Autodesk Fusion 360 part; units mm, degrees
sketch "Sketch1" plane through (0, 0, 0) normal (1, 0, 0) x (0, 1, 0)
  line L0 (0, 0) -> (15, 0) construction
  line L1 (15, 0) -> (15, 4.5) construction
  circle A0 centre (15, 4.5) radius 3
  line L2 (15, 0) -> (11, 0) construction
  line L3 (11, 0) -> (19, 0)
  line L4 (19, 0) -> (19, 3.75)
  line L5 (19, 3.75) -> (11, 3.75)
  line L6 (11, 3.75) -> (2.6, 3.75)
  line L7 (2.6, 3.75) -> (2.6, 0)
  line L8 (2.6, 0) -> (11, 0)
  dimension "d1" = 15
  dimension "d2" = 4.5
  dimension "d3" = 6
  dimension "d4" = 4
  dimension "d5" = 8
  dimension "d6" = 3.75
  dimension "d7" = 2.6
revolve "Revolve1" add sketch "Sketch1" angle 360 about axis through (0, 0, 1.75) along (0, 0, 1) contours A0 L3 L4 L5 L6 L7 L8
fillet "Fillet1" radius 1.5 1 edges at (-17.7142, 6.8707, 0)
Input: part model. Units: mm. Frame: model coordinates. Give positions to 0.01 mm unless a question says otherwise; leave off trailing zeros. Order: outer loops, then holes, each group sorted by start corner. A loop starts at its lowest first (then second) coordinate and runs counter-clockwise, first axis right, second up.
Q1. Section A-A on y = 0. Output: boundary loops of the cut face in (x, z).
Checked values:
outline: (-19, 1.5) arc R1.5 ccw to (-17.5, 0) - (-2.6, 0) - (-2.6, 3.75) - (-12.1, 3.75) arc R3 cw to (-17.9, 3.75) - (-19, 3.75) - close; (2.6, 0) - (17.5, 0) arc R1.5 ccw to (19, 1.5) - (19, 3.75) - (17.9, 3.75) arc R3 cw to (12.1, 3.75) - (2.6, 3.75) - close
Q2. Contact query for a flat-ended pin moving along its axis: pin 1 Ø1.5 at (y, z) = (-14.5, 2.5) entering from -X. Output: stop coordinate, or through.
Checked values:
pin 1: stops at x = -13.11
Q3. Section D-D on z = 0.9. Output: boundary loops of the cut face in (x, y).
Checked values:
outline: circle Ø37.75 at (0, 0); hole circle Ø5.2 at (0, 0)
Q4. Section C-C on z = 2.95. Output: boundary loops of the cut face in (x, y).
Checked values:
outline: circle Ø38 at (0, 0); circle Ø24.86 at (0, 0); hole circle Ø35.14 at (0, 0); hole circle Ø5.2 at (0, 0)
Q5. Ray query, probe 1 along Y at (x, z) = (0, 2.9); probe 2 along Y at (x, z) = (0, 2.75); probe 3 along X at (y, z) = (-9.5, 2.95). Return the intervals inside material, ascending.
Checked values:
probe 1: y = -19 to -17.54, -12.46 to -2.6, 2.6 to 12.46, 17.54 to 19
probe 2: y = -19 to -17.44, -12.56 to -2.6, 2.6 to 12.56, 17.44 to 19
probe 3: x = -16.45 to -14.78, -8.02 to 8.02, 14.78 to 16.45
Q6. Draft query along Y for faces 1 (the cylindrical face through (2.578, -0.338, 1.849)), 2 (the cylindrical face through (16.856, 8.767, 2.641)), 3 (the flat face through (0, -3, 3.75)). Return one class per face: +Y half, -Y half, draft (parallel to the pull), parting line (faces both ways), or undercut.
Checked values:
face 1: undercut
face 2: parting line
face 3: draft
